Autodesk Inventor part; units mm, degrees
ref_plane "YZ Plane" through (0, 0, 0) normal (1, 0, 0) x (0, 1, 0)
ref_plane "XZ Plane" through (0, 0, 0) normal (0, 1, 0) x (-1, 0, 0)
ref_plane "XY Plane" through (0, 0, 0) normal (0, 0, 1) x (1, 0, 0)
sketch "Sketch1" plane through (0, 0, 0) normal (0, 0, 1) x (1, 0, 0)
  line L0 (0, 0) -> (0, -38.05)
  line L1 (0, -38.05) -> (3.175, -38.05)
  line L2 (3.175, -38.05) -> (3.175, 0)
  line L3 (3.175, 0) -> (0, 0)
  line L4 (3.175, 0) -> (3.175, -6.85)
  line L5 (3.175, -6.85) -> (12.025, -6.85)
  line L6 (12.025, -6.85) -> (12.025, 0)
  line L7 (12.025, 0) -> (15.2, 0)
  line L8 (15.2, 0) -> (15.2, -6.85)
  line L9 (15.2, -6.85) -> (15.2, -8.85)
  line L10 (15.2, -8.85) -> (3.175, -8.85)
  line L11 (0, -38.05) -> (0, -31.2)
  dimension "d0" = 38.05
  dimension "d1" = 3.175
  dimension "d2" = 6.85
  dimension "d3" = 8.85
  dimension "d4" = 3.175
  dimension "d5" = 2
extrude "Extrusion1" add sketch "Sketch1" along normal blind 49.213
sketch "Sketch2" plane through (0, 0, 0) normal (0, 0, -1) x (-1, 0, 0)
  line L0 (0, -38.05) -> (-3.175, -38.05)
  line L1 (0, -38.05) -> (0, -32.05)
  line L2 (0, 0) -> (0, -38.05)
  line L3 (0, -32.05) -> (0, -23.25)
  line L4 (0, -23.25) -> (6.6, -23.25)
  line L5 (6.6, -23.25) -> (6.6, -32.05)
  line L6 (6.6, -32.05) -> (0, -32.05)
  dimension "d12" = 6
  dimension "d13" = 8.8
  dimension "d14" = 6.6
extrude "Extrusion2" add sketch "Sketch2" against normal blind 3.175
sketch "Sketch3" plane through (0, 0, 3.175) normal (0, 0, 1) x (1, 0, 0)
  line L0 (0, -23.25) -> (0, -32.05)
  line L1 (0, -23.25) -> (-3.3, -23.25)
  line L2 (0, -23.25) -> (-6.6, -23.25)
  line L3 (-3.3, -23.25) -> (-3.3, -27.65)
  point P0 (0, 0)
  dimension "d17" = 4.4
hole "Hole1" at (-3.3, -27.65, 3.175) direction (0, 0, -1) diameter 3 end through all
fillet "Fillet1" radius 2 2 edges at (-6.6, -23.25, 1.5875) (-6.6, -32.05, 1.5875)
sketch "Sketch4" plane through (0, 0, 49.213) normal (0, 0, 1) x (1, 0, 0)
  line L0 (3.175, 0) -> (0, 0)
  line L1 (3.175, -8.85) -> (15.2, -8.85)
  line L2 (0, 0) -> (15.2, 0)
  line L3 (15.2, 0) -> (15.2, -8.85)
  line L4 (15.2, -8.85) -> (0, -8.85)
  line L5 (0, -8.85) -> (0, 0)
extrude "Extrusion3" add sketch "Sketch4" along normal blind 1.5875
sketch "Sketch5" plane through (0, 0, 50.8005) normal (0, 0, 1) x (1, 0, 0)
  line L0 (3.175, 0) -> (0, 0)
  line L1 (0, 0) -> (3.175, 0)
  line L2 (3.175, 0) -> (12.025, 0)
  line L3 (3.175, 0) -> (7.6, 0)
  line L4 (7.6, 0) -> (7.6, -3.425)
  dimension "d28" = 3.425
hole "Hole2" at (7.6, -3.425, 50.8005) direction (0, 0, -1) diameter 3 end through all
fillet "Fillet2" radius 2 2 edges at (0, -8.85, 50.0068) (15.2, -8.85, 25.4003)
sketch "Sketch6" plane through (0, -38.05, 0) normal (-1, 0, 0) x (0, 0, 1)
  line L0 (0, 0) -> (0, 29.2)
  line L1 (0, 0) -> (0, 28.2)
  line L2 (0, 28.2) -> (28.2, 28.2)
  line L3 (28.2, 28.2) -> (28.2, 0)
  line L4 (0, 0) -> (49.213, 0)
  line L5 (0, 0) -> (0, 14.1)
  line L6 (0, 12.8) -> (0, 14.8)
  line L7 (0, 14.1) -> (14.1, 14.1)
  line L8 (14.1, 14.1) -> (2.6, 14.1)
  line L9 (2.6, 14.1) -> (2.6, 2.6)
  line L10 (0, 12.8) -> (3.175, 12.8)
  line L11 (2.6, 2.6) -> (25.6, 2.6)
  line L12 (25.6, 2.6) -> (25.6, 25.6)
  line L13 (25.6, 25.6) -> (2.6, 25.6)
  line L14 (2.6, 25.6) -> (2.6, 2.6)
  point P0 (0, 38.05)
  dimension "d37" = 28.2
  dimension "d38" = 28.2
  dimension "d39" = 11.5
  dimension "d40" = 11.5
  dimension "d41" = 90
  dimension "d42" = 23
  dimension "d43" = 23
hole "Hole3" at (0, -35.45, 2.6) at (0, -35.45, 25.6) at (0, -12.45, 25.6) at (0, -12.45, 2.6) direction (1, 0, 0) diameter 2.5 end through all
delete faces "Delete1" heal yes whole lump no faces at (7.7207, -4.9201, 50.2713)
sketch "Sketch7" plane through (0, 0, 50.8005) normal (0, 0, 1) x (1, 0, 0)
  line L0 (15.2, -6.85) -> (15.2, 0)
  line L1 (15.2, 0) -> (0, 0)
  line L2 (15.2, 0) -> (0, 0)
  line L3 (0, 0) -> (7.6, 0)
  line L4 (7.6, 0) -> (7.6, -2.15)
  dimension "d51" = 2.15
hole "Hole4" at (7.6, -2.15, 50.8005) direction (0, 0, -1) diameter 3 depth 3.5
sketch "Sketch8" plane through (0, 0, 49.213) normal (0, 0, 1) x (1, 0, 0)
  line L0 (0, -38.05) -> (3.175, -38.05)
  line L1 (3.175, -38.05) -> (0, -38.05)
  line L2 (3.175, -23.45) -> (0, -23.45)
  line L3 (0, -23.45) -> (0, -17.45)
  line L4 (0, -17.45) -> (3.175, -17.45)
  line L5 (3.175, -17.45) -> (3.175, -23.45)
  line L6 (3.175, -23.45) -> (0, -23.45)
  line L7 (0, -23.45) -> (0, -29.45)
  line L8 (0, -29.45) -> (3.175, -29.45)
  line L9 (3.175, -29.45) -> (3.175, -23.45)
  point P0 (0, 0)
  point P1 (3.175, -8.85)
  dimension "d59" = 6
  dimension "d60" = 6
extrude "Extrusion4" cut sketch "Sketch8" against normal blind 3.175
fillet "Fillet3" radius 2 2 edges at (1.5875, -17.45, 46.038) (1.5875, -29.45, 46.038)
sketch "Sketch9" plane through (0, 0, 46.038) normal (0, 0, 1) x (1, 0, 0)
  line L0 (3.175, -17.45) -> (0, -17.45)
  line L1 (0, -29.45) -> (3.175, -29.45)
  line L2 (0, -17.45) -> (3.175, -17.45)
  line L3 (3.175, -17.45) -> (3.175, -29.45)
  line L4 (3.175, -29.45) -> (0, -29.45)
  line L5 (0, -29.45) -> (0, -17.45)
  point P0 (0, 0)
extrude "Extrusion5" add sketch "Sketch9" along normal blind 3.175
delete faces "Delete Face1" heal yes whole lump no faces at (1.0583, -12.3494, 3.8459) (1.0583, -12.3494, 26.8459) (1.0583, -35.3494, 26.8459) (1.0583, -35.3494, 3.8459)
sketch "Sketch10" plane through (0, -38.05, 0) normal (0, -1, 0) x (1, 0, 0)
  line L0 (3.175, 0) -> (3.175, 49.213)
  line L1 (3.175, 49.213) -> (3.175, 45.048)
  line L2 (3.175, 45.048) -> (6.6749, 17.1164)
  line L3 (6.6749, 17.1164) -> (3.175, 16.6779)
  line L4 (3.175, 16.6779) -> (3.175, 45.048)
  point P0 (0, 0)
  dimension "d66" = 4.165
  dimension "d67" = 28.15
  dimension "d68" = 172.858
extrude "Extrusion6" add sketch "Sketch10" against normal up to next
sketch "Sketch11" plane through (3.175, -38.05, 45.048) normal (0.9922411, 0, 0.1243289) x (0.1243289, 0, -0.9922411)
  line L0 (44.6985, 29.2) -> (28.15, 29.2)
  line L1 (0, 0) -> (28.15, 29.2)
  line L2 (0, 0) -> (0, 29.2)
  line L3 (28.15, 0) -> (28.15, 29.2)
  line L4 (0, 29.2) -> (28.15, 0)
  line L5 (14.075, 14.6) -> (2.575, 14.6)
  line L6 (2.575, 14.6) -> (2.575, 26.1)
  line L7 (2.575, 26.1) -> (14.075, 26.1)
  line L8 (14.075, 26.1) -> (14.075, 14.6)
  line L9 (14.075, 14.6) -> (2.575, 14.6)
  line L10 (2.575, 14.6) -> (2.575, 3.1)
  line L11 (2.575, 3.1) -> (14.075, 3.1)
  line L12 (14.075, 3.1) -> (14.075, 14.6)
  line L13 (14.075, 14.6) -> (25.575, 14.6)
  line L14 (25.575, 14.6) -> (25.575, 3.1)
  line L15 (25.575, 3.1) -> (14.075, 3.1)
  line L16 (14.075, 3.1) -> (14.075, 14.6)
  line L17 (14.075, 14.6) -> (25.575, 14.6)
  line L18 (25.575, 14.6) -> (25.575, 26.1)
  line L19 (25.575, 26.1) -> (14.075, 26.1)
  line L20 (14.075, 26.1) -> (14.075, 14.6)
  point P0 (44.3037, 38.05)
  dimension "d71" = 11.5
  dimension "d72" = 11.5
  dimension "d73" = 11.5
  dimension "d74" = 11.5
  dimension "d75" = 11.5
  dimension "d76" = 11.5
  dimension "d77" = 11.5
  dimension "d78" = 11.5
hole "Hole5" at (3.4951, -34.95, 42.493) at (3.4951, -11.95, 42.493) at (6.3547, -11.95, 19.6714) at (6.3547, -34.95, 19.6714) direction (-0.9922411, 0, -0.1243289) diameter 2.75 end through all
sketch "Sketch12" plane through (0, -38.05, 0) normal (0, -1, 0) x (1, 0, 0)
  line L0 (3.175, 45.048) -> (6.6749, 17.1164)
  line L1 (6.6749, 17.1164) -> (3.175, 11.0545)
  line L2 (3.175, 49.213) -> (3.175, 0)
  line L3 (6.6749, 17.1164) -> (13.6746, 17.1164) construction
  line L4 (3.175, 11.0545) -> (3.175, 16.6739)
  line L5 (6.6749, 17.1164) -> (3.175, 16.6779)
  line L6 (6.6749, 17.1164) -> (3.175, 16.6779)
  point P0 (0, 0)
  dimension "d86" = 120
extrude "Extrusion7" add sketch "Sketch12" against normal up to next contours L1 L2 L5
sketch "Sketch13" plane through (0, -38.05, 0) normal (0, -1, 0) x (1, 0, 0)
  line L0 (3.175, 45.048) -> (6.6749, 17.1164)
  line L1 (3.175, 45.048) -> (0, 45.048)
  line L2 (0, 0) -> (0, 50.8005)
  line L3 (6.6749, 17.1164) -> (0, 17.1164)
  line L4 (6.6749, 17.1164) -> (3.4999, 17.1164)
  line L5 (3.4999, 17.1164) -> (0, 45.048)
  line L6 (3.4999, 17.1164) -> (0, 11.0545)
  line L7 (3.4999, 17.1164) -> (10.4996, 17.1164) construction
  line L8 (0, 11.0545) -> (0, 45.048)
  dimension "d89" = 3.175
  dimension "d90" = 120
extrude "Extrusion8" cut sketch "Sketch13" against normal up to surface (29.2 mm away) contours L5 L3 L2 | L6 L2 L3
sketch "Sketch14" plane through (3.175, -38.05, 0) normal (1, 0, 0) x (0, 0, -1)
  point P0 (0, 38.05)
sketch "Sketch15" plane through (3.175, -38.05, 0) normal (1, 0, 0) x (0, 0, -1)
  line L0 (0, 29.2) -> (-11.0545, 29.2)
  line L1 (0, 14.8) -> (-3.175, 14.8)
  line L2 (0, 29.2) -> (0, 14.8)
  line L3 (0, 14.8) -> (0, 22)
  line L4 (0, 0) -> (0, 29.2)
  line L5 (0, 22) -> (0, 28)
  line L6 (0, 28) -> (-6, 28)
  line L7 (-6, 28) -> (-6, 16)
  line L8 (-6, 16) -> (0, 16)
  line L9 (0, 16) -> (0, 28)
  point P0 (0, 38.05)
  dimension "d93" = 7.2
  dimension "d94" = 6
  dimension "d95" = 6
  dimension "d96" = 12
extrude "Extrusion9" cut sketch "Sketch15" against normal up to next
fillet "Fillet4" radius 2 2 edges at (1.5875, -22.05, 6) (1.5875, -10.05, 6)
properties part number "Yaw Motor Mount_v2"
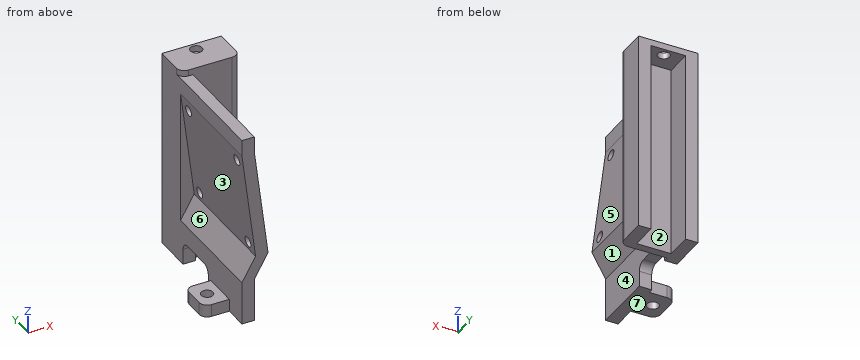
Part model, mm, in its own coordinate system. Face numbers are marked on the shaded views. A direction names the side the tool comes from. Coordinates: 2 decimals unless noted, no trailing zeros. Loops run counter-clockwise (first coordinate to the right, second up) from the corner with the lowest first, then second, coordinate; pieces in that order, holes last. Notation, with made-up numbers: M 59.25,69 L 68.25,69 A23 ccw 68.25,85 Z; hole C 64.5,44 d2. An arc over 180 degrees is marked long. Use a Markdown table: item, result. Add a question column.
Q1. Cut at A-A (y = -27.65). Write the cut outline in (x, z) (1 decimal).
Q2. Which spindle directions (+Z, -Z, +X, -X, +Y, -Y) get a long thin tool onto all of the face, cutting with end or side? Do the marked faces 4, 5, 6 and 7. Say none if no direction does.
Q3. Pin check, flat tips, straight feed: P1, Ø3.5, axis at x = 7.6, y = -2.15, coming from the +Z side; P2, Ø12, axis at y = -34, z = 27.5, coming from the +X side; P3, Ø1, axis at x = 6, z = 6.5, coming from the +Y side; P4, Ø5.5, axis at y = -25.5, z = 5, coming from the +X side (3 decimals). Stop position of each tip, or through.
Q4. Cut at B-B (x = -3.3). Write the cut outline in (y, z) (3 decimals), and give its area (3 significant figures).
Q5. Probe L1, parallel to Y at x = -3.3, z = 1.45; L2, parallel to Z at x = -5.5, y = -25 (3 decimals); L3, parallel to Y at x = 1, z = 2. List the from-to ranges inside material, lowest first.
Q6. Cut at D-D (z = 23.5). Write the cut outline in (x, y) (3 decimals), and give its area (3 significant figures).
Q7. Mould opens along X. For the marked faces 1, 2 and 3 say: +X half, -X half, draft (parallel to the pull), parting line (faces both ways), or undercut.
Q8. Cut at C-C (y = -33). Write the cut outline in (x, z) (1 decimal).
Worked out:
| question | item | result |
|---|---|---|
| 1 | outline | M -6.6,0 L -4.8,0 L -4.8,3.2 L -6.6,3.2 Z; M -1.8,0 L 3.2,0 L 3.2,11.1 L 6.7,17.1 L 3.2,45 L 3.2,49.2 L 0,49.2 L 0,45 L 3.5,17.1 L 0,11.1 L 0,3.2 L -1.8,3.2 Z |
| 2 | face 4 | -Z, +X, -Y |
| 2 | face 5 | +Z, +X, -Y |
| 2 | face 6 | -X, -Y |
| 2 | face 7 | -Z, +X, -X, +Y, -Y |
| 3 | P1 | stops at z = 50.8 |
| 3 | P2 | stops at x = 6.13 |
| 3 | P3 | stops at y = -6.85 |
| 3 | P4 | stops at x = 3.175 |
| 4 | outline | M -32.05,0 L -29.15,0 L -29.15,3.175 L -32.05,3.175 Z; M -26.15,0 L -23.25,0 L -23.25,3.175 L -26.15,3.175 Z |
| 4 | area | 18.4 mm2 |
| 5 | L1 | y = -32.05 to -29.15, -26.15 to -23.25 |
| 5 | L2 | z = 0 to 3.175 |
| 5 | L3 | y = -38.05 to -22.05, -10.05 to 0 |
| 6 | outline | M 0,-8.85 L 2.7,-8.85 L 2.7,-38.05 L 5.875,-38.05 L 5.875,-8.85 L 13.2,-8.85 A2 ccw 15.2,-6.85 L 15.2,0 L 12.025,0 L 12.025,-6.85 L 3.175,-6.85 L 3.175,0 L 0,0 Z |
| 6 | area | 166 mm2 |
| 7 | face 1 | +X half |
| 7 | face 2 | undercut |
| 7 | face 3 | -X half |
| 8 | outline | M 0,0 L 3.2,0 L 3.2,11.1 L 6.7,17.1 L 3.2,45 L 3.2,49.2 L 0,49.2 L 0,45 L 3.5,17.1 L 0,11.1 Z |
